Read the model definition and answer for the solid it produces. Units are mm, in the model's axes. Face numbers are marked on the shaded views. A direction names the side the tool comes from. Coordinates: 2 decimals unless noted, no trailing zeros. Write each loop counter-clockwise with the first axis right and the second up, starting at its lowest first coordinate (ties: lowest second). Pieces come first, ordered by that corner, then holes.
(1) Find the intervals of material crossed by probe 1 along Y at (x, z) = (0, 1.2); probe 2 along Y at (x, z) = (-5, 4.5); probe 3 along X at (y, z) = (-5, 7.75), in increasing order.
(2) Given pin 1 (10 mm diameter, centred on x = -1, y = 6, fed in from +Z); pin 2 (6 mm diameter, centred on x = -0.5, y = 3, fed in from +Z); pin 3 (9.5 mm diameter, centred on x = -4, y = -3.5, fed in from +Z), each flat-ended and moving along its own axis, determine where each tip first touches the part or whether it passes through.
(3) Section A-A on y = 0 is taken. Write down the section's boundary in (x, z), then the cut area to 3 significant figures.
(4) Section B-B on z = 4.5 is taken. Write down the section's boundary in (x, y).
(5) The mould has two halves that part along X. Classify the marked faces 3, 4 and 5: +X half, -X half, draft (parallel to the pull), parting line (faces both ways), or undercut.
(6) Which of the six approach directions +Z, -Z, +X, -X, +Y, -Y give full straight-line access (tool end or side, diameter ignored) to the marked faces 1 and 2?
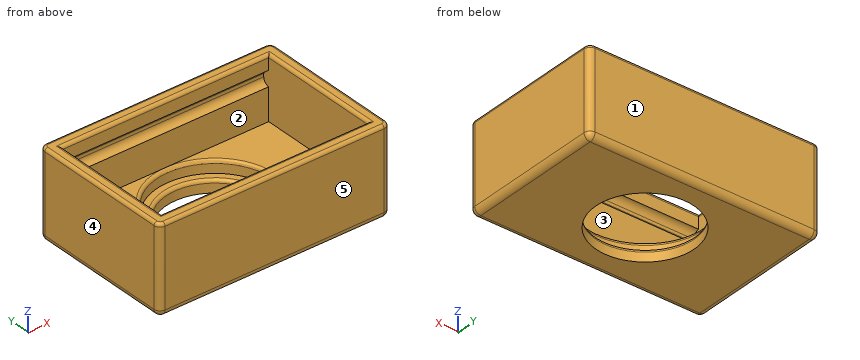
from build123d import *

# Parameters (mm, degrees)
F0_W          = 37.8
F0_H          = 24
F0_W_2        = 33.8
F0_H_2        = 20
F1_DEPTH      = 14.2
F0_R          = 9.5
F2_DEPTH      = 4
F0_R_2        = 8
F3_DEPTH      = 2
F4_W          = 33.8
F4_H          = 2.5
F5_DEPTH      = 1
F7_DEPTH      = 1
F8_R          = 0.49999
F9_R          = 0.99999
F10_T1_DEPTH  = 35.8
F10_T3_DEPTH  = 22
F10_T5_DEPTH  = 13.2
F10_T8_ANGLE  = 90
F10_T10_ANGLE = 90
F10_T12_ANGLE = 90
F10_T14_ANGLE = 90
F10_S17_W     = 1
F10_S17_H     = 1
F10_T18_DEPTH = 1
F10_S23_W     = 1
F10_S23_H     = 1
F10_T24_DEPTH = 1
F10_S29_W     = 1
F10_S29_H     = 1
F10_T30_DEPTH = 1
F10_S35_W     = 1
F10_S35_H     = 1
F10_T36_DEPTH = 1


# Not quite as in the source:
# - a fillet or chamfer that OpenCascade refuses, or shapes differently, is made with other operations: its cross-section is extruded or revolved along the edge and cut away or added
# - a fillet or chamfer is up to 0.001 mm smaller than in the source, because OpenCascade refuses the exact size


with BuildPart() as f1:
    # F0 (on Top) → F1 (new body)
    with BuildSketch(Plane.XY):
        Rectangle(F0_W, F0_H)
        Rectangle(F0_W_2, F0_H_2, mode=Mode.SUBTRACT)
    extrude(amount=F1_DEPTH)

    # F0 (on Top) → F2 (join)
    with BuildSketch(Plane.XY):
        Rectangle(F0_W_2, F0_H_2)
        Circle(F0_R, mode=Mode.SUBTRACT)
    extrude(amount=F2_DEPTH)

    # F0 (on Top) → F3 (join)
    with BuildSketch(Plane.XY):
        Circle(F0_R)
        Circle(F0_R_2, mode=Mode.SUBTRACT)
    extrude(amount=F3_DEPTH)

    # F4 (on face) → F5 (cut)
    with BuildSketch(Plane.XZ.offset(-10)):
        with Locations((0, 10.55)):
            Rectangle(F4_W, F4_H)
    extrude(amount=-F5_DEPTH, mode=Mode.SUBTRACT)

    # F6 (on face) → F7 (cut)
    with BuildSketch(Plane(origin=(0, -10, 0), x_dir=(-1, 0, 0), z_dir=(0, 1, 0))):
        Polygon((-16.9, 9.3), (1.5624057269, 9.3), (16.9, 9.3), (16.9, 11.8), (-16.9, 11.8), align=None)
    extrude(amount=-F7_DEPTH, mode=Mode.SUBTRACT)

    # F8 (radius 0.5 in the source; OpenCascade refuses exactly that, so slightly less here)
    f8_edges = [f1.edges().sort_by_distance(p)[0] for p in [
        (-9.5, 0, 4),
        (-8, 0, 2),
        (0, 10, 14.2),
        (16.9, 0, 14.2),
        (-16.9, 0, 14.2),
        (0, -10, 14.2),
        (0, -12, 14.2),
        (18.9, 0, 14.2),
        (0, 12, 14.2),
        (-18.9, 0, 14.2),
    ]]
    fillet(f8_edges, radius=F8_R)

    # F9 (radius 1 in the source; OpenCascade refuses exactly that, so slightly less here)
    f9_edges = [f1.edges().sort_by_distance(p)[0] for p in [
        (0, 11, 9.3),
        (0, 11, 11.8),
        (0, -11, 9.3),
        (0, -11, 11.8),
    ]]
    fillet(f9_edges, radius=F9_R)

    # F10: fillet of radius 1 on 8 edges, made by hand

    # F10_s2 → F10_t1 (cut)
    with BuildSketch(Plane.YZ.offset(-17.9)):
        with BuildLine():
            ThreePointArc((-12, 1), (-11.7071067812, 0.2928932188), (-11, 0))
            Line((-11, 0), (-12, 0))
            Line((-12, 0), (-12, 1))
        make_face()
        with BuildLine():
            ThreePointArc((12, 1), (11.7071067812, 0.2928932188), (11, 0))
            Line((11, 0), (12, 0))
            Line((12, 0), (12, 1))
        make_face()
    extrude(amount=F10_T1_DEPTH, mode=Mode.SUBTRACT)

    # F10_s4 → F10_t3 (cut)
    with BuildSketch(Plane.XZ.offset(-11)):
        with BuildLine():
            ThreePointArc((-18.9, 1), (-18.6071067812, 0.2928932188), (-17.9, 0))
            Line((-17.9, 0), (-18.9, 0))
            Line((-18.9, 0), (-18.9, 1))
        make_face()
        with BuildLine():
            ThreePointArc((18.9, 1), (18.6071067812, 0.2928932188), (17.9, 0))
            Line((17.9, 0), (18.9, 0))
            Line((18.9, 0), (18.9, 1))
        make_face()
    extrude(amount=F10_T3_DEPTH, mode=Mode.SUBTRACT)

    # F10_s6 → F10_t5 (cut)
    with BuildSketch(Plane.XY.offset(1)):
        with BuildLine():
            ThreePointArc((17.9, -12), (18.6071067812, -11.7071067812), (18.9, -11))
            Line((18.9, -11), (18.9, -12))
            Line((18.9, -12), (17.9, -12))
        make_face()
        with BuildLine():
            ThreePointArc((-17.9, -12), (-18.6071067812, -11.7071067812), (-18.9, -11))
            Line((-18.9, -11), (-18.9, -12))
            Line((-18.9, -12), (-17.9, -12))
        make_face()
        with BuildLine():
            ThreePointArc((18.9, 11), (18.6071067812, 11.7071067812), (17.9, 12))
            Line((17.9, 12), (18.9, 12))
            Line((18.9, 12), (18.9, 11))
        make_face()
        with BuildLine():
            ThreePointArc((-18.9, 11), (-18.6071067812, 11.7071067812), (-17.9, 12))
            Line((-17.9, 12), (-18.9, 12))
            Line((-18.9, 12), (-18.9, 11))
        make_face()
    extrude(amount=F10_T5_DEPTH, mode=Mode.SUBTRACT)

    # F10_s7 → F10_t8 (revolve, cut)
    with BuildSketch(Plane.YZ.offset(-17.9)):
        with BuildLine():
            ThreePointArc((11.50001, 14.2), (11.8535563195, 14.0535563195), (12, 13.70001))
            Line((12, 13.70001), (12, 14.2))
            Line((12, 14.2), (11.50001, 14.2))
        make_face()
    revolve(axis=Axis((-17.9, 11, 14.2), (0, 0, 1)), revolution_arc=F10_T8_ANGLE, mode=Mode.SUBTRACT)

    # F10_s9 → F10_t10 (revolve, cut)
    with BuildSketch(Plane.XZ.offset(-11)):
        with BuildLine():
            ThreePointArc((18.40001, 14.2), (18.7535563195, 14.0535563195), (18.9, 13.70001))
            Line((18.9, 13.70001), (18.9, 14.2))
            Line((18.9, 14.2), (18.40001, 14.2))
        make_face()
    revolve(axis=Axis((17.9, 11, 14.2), (0, 0, 1)), revolution_arc=F10_T10_ANGLE, mode=Mode.SUBTRACT)

    # F10_s11 → F10_t12 (revolve, cut)
    with BuildSketch(Plane.XZ.offset(11)):
        with BuildLine():
            ThreePointArc((-18.40001, 14.2), (-18.7535563195, 14.0535563195), (-18.9, 13.70001))
            Line((-18.9, 13.70001), (-18.9, 14.2))
            Line((-18.9, 14.2), (-18.40001, 14.2))
        make_face()
    revolve(axis=Axis((-17.9, -11, 14.2), (0, 0, 1)), revolution_arc=F10_T12_ANGLE, mode=Mode.SUBTRACT)

    # F10_s13 → F10_t14 (revolve, cut)
    with BuildSketch(Plane.YZ.offset(17.9)):
        with BuildLine():
            ThreePointArc((-11.50001, 14.2), (-11.8535563195, 14.0535563195), (-12, 13.70001))
            Line((-12, 13.70001), (-12, 14.2))
            Line((-12, 14.2), (-11.50001, 14.2))
        make_face()
    revolve(axis=Axis((17.9, -11, 14.2), (0, 0, 1)), revolution_arc=F10_T14_ANGLE, mode=Mode.SUBTRACT)


with BuildPart() as f10_tool16:
    # F10_s17 → F10_t18 (new body)
    with BuildSketch(Plane.XY.offset(1)):
        with Locations((-18.4, -11.5)):
            Rectangle(F10_S17_W, F10_S17_H)
    extrude(amount=-F10_T18_DEPTH)

    # F10_s19 → F10_t20 (revolve, cut)
    with BuildSketch(Plane(origin=(-17.9, -11, 1), x_dir=(0.7071067812, 0.7071067812, 0), z_dir=(-0.7071067812, 0.7071067812, 0))):
        with BuildLine():
            ThreePointArc((0, -1), (1, 0), (0, 1))
            Line((0, 1), (0, -1))
        make_face()
    revolve(axis=Axis((-17.9, -11, 1), (0, 0, -1)), mode=Mode.SUBTRACT)


with BuildPart() as f1_1:
    add(f1.part)

    # F10_t15: cut F10_tool16
    add(f10_tool16.part, mode=Mode.SUBTRACT)


with BuildPart() as f10_tool22:
    # F10_s23 → F10_t24 (new body)
    with BuildSketch(Plane.XY.offset(1)):
        with Locations((18.4, -11.5)):
            Rectangle(F10_S23_W, F10_S23_H)
    extrude(amount=-F10_T24_DEPTH)

    # F10_s25 → F10_t26 (revolve, cut)
    with BuildSketch(Plane(origin=(17.9, -11, 1), x_dir=(-0.7071067812, 0.7071067812, 0), z_dir=(-0.7071067812, -0.7071067812, 0))):
        with BuildLine():
            ThreePointArc((0, -1), (1, 0), (0, 1))
            Line((0, 1), (0, -1))
        make_face()
    revolve(axis=Axis((17.9, -11, 1), (0, 0, -1)), mode=Mode.SUBTRACT)


with BuildPart() as f1_2:
    add(f1_1.part)

    # F10_t21: cut F10_tool22
    add(f10_tool22.part, mode=Mode.SUBTRACT)


with BuildPart() as f10_tool28:
    # F10_s29 → F10_t30 (new body)
    with BuildSketch(Plane.XY.offset(1)):
        with Locations((-18.4, 11.5)):
            Rectangle(F10_S29_W, F10_S29_H)
    extrude(amount=-F10_T30_DEPTH)

    # F10_s31 → F10_t32 (revolve, cut)
    with BuildSketch(Plane(origin=(-17.9, 11, 1), x_dir=(0.7071067812, -0.7071067812, 0), z_dir=(0.7071067812, 0.7071067812, 0))):
        with BuildLine():
            ThreePointArc((0, -1), (1, 0), (0, 1))
            Line((0, 1), (0, -1))
        make_face()
    revolve(axis=Axis((-17.9, 11, 1), (0, 0, -1)), mode=Mode.SUBTRACT)


with BuildPart() as f1_3:
    add(f1_2.part)

    # F10_t27: cut F10_tool28
    add(f10_tool28.part, mode=Mode.SUBTRACT)


with BuildPart() as f10_tool34:
    # F10_s35 → F10_t36 (new body)
    with BuildSketch(Plane.XY.offset(1)):
        with Locations((18.4, 11.5)):
            Rectangle(F10_S35_W, F10_S35_H)
    extrude(amount=-F10_T36_DEPTH)

    # F10_s37 → F10_t38 (revolve, cut)
    with BuildSketch(Plane(origin=(17.9, 11, 1), x_dir=(-0.7071067812, -0.7071067812, 0), z_dir=(0.7071067812, -0.7071067812, 0))):
        with BuildLine():
            ThreePointArc((0, -1), (1, 0), (0, 1))
            Line((0, 1), (0, -1))
        make_face()
    revolve(axis=Axis((17.9, 11, 1), (0, 0, -1)), mode=Mode.SUBTRACT)


with BuildPart() as f1_4:
    add(f1_3.part)

    # F10_t33: cut F10_tool34
    add(f10_tool34.part, mode=Mode.SUBTRACT)


solid = f1_4.part
Response:
1. probe 1: y = -12 to -8, 8 to 12
1. probe 2: y = -12 to -10, 10 to 12
1. probe 3: x = -18.9 to -16.9, 16.9 to 18.9
2. pin 1: stops at z = 14.2
2. pin 2: passes through
2. pin 3: stops at z = 4
3. outline: (-18.9, 1) arc R1 ccw to (-17.9, 0) - (-8, 0) - (-8, 1.5) arc R0.5 ccw to (-8.5, 2) - (-9.5, 2) - (-9.5, 3.5) arc R0.5 ccw to (-10, 4) - (-16.9, 4) - (-16.9, 13.7) arc R0.5 ccw to (-17.4, 14.2) - (-18.4, 14.2) arc R0.5 ccw to (-18.9, 13.7) - close; (8, 0) - (17.9, 0) arc R1 ccw to (18.9, 1) - (18.9, 13.7) arc R0.5 ccw to (18.4, 14.2) - (17.4, 14.2) arc R0.5 ccw to (16.9, 13.7) - (16.9, 4) - (10, 4) arc R0.5 ccw to (9.5, 3.5) - (9.5, 2) - (8.5, 2) arc R0.5 ccw to (8, 1.5) - close
3. area: 121 mm2
4. outline: (-18.9, -11) arc R1 ccw to (-17.9, -12) - (17.9, -12) arc R1 ccw to (18.9, -11) - (18.9, 11) arc R1 ccw to (17.9, 12) - (-17.9, 12) arc R1 ccw to (-18.9, 11) - close; hole (-16.9, -10) - (16.9, -10) - (16.9, 10) - (-16.9, 10) - close
5. face 3: undercut
5. face 4: -X half
5. face 5: draft
6. face 1: +Z, -Z, +X, -X, +Y
6. face 2: +Z
